Input: dimensioned drawing with shaded views. Units: mm. Origin: part minimum x, y, z. A direction names the side the tool comes from. Give positions to 0.01 mm unless a question says otherwise; leave off trailing zeros. Loops run counter-clockwise (first coordinate to the right, second up) from the corner with the lowest first, then second, coordinate; pieces in that order, holes last. Notation, with made-up numbers: (-19, 9) -> (16, 9) arc R21 cw to (16, 15) -> close; hole circle Ø7 at (-11, 32). An arc over 180 degrees is marked (long way). Answer as a JSON object with one key per item and string values.
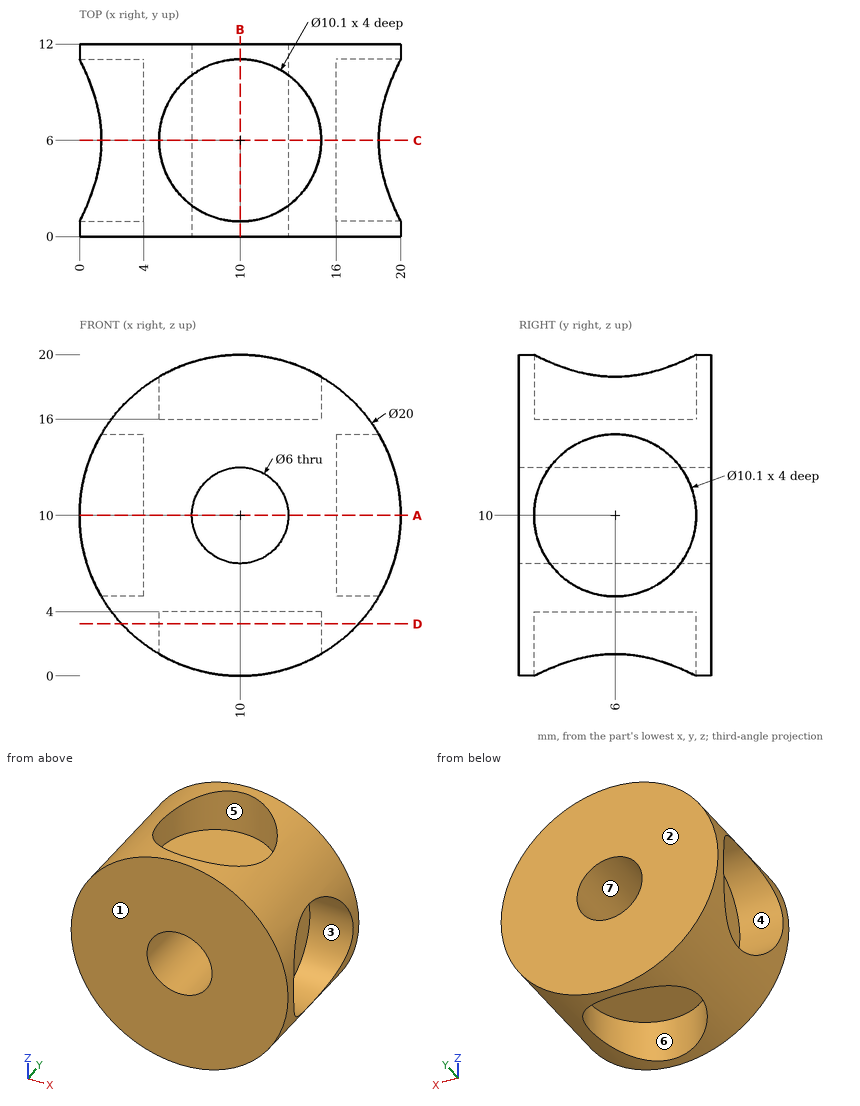
Q1. Section C-C, the plane y = 6. Return the cut outline in (x, z), then the cut area to 3 significant figures.
Evaluation:
{"outline": "(1.37, 4.95) arc R10 ccw to (4.95, 1.37) -> (4.95, 4) -> (15.05, 4) -> (15.05, 1.37) arc R10 ccw to (18.63, 4.95) -> (16, 4.95) -> (16, 15.05) -> (18.63, 15.05) arc R10 ccw to (15.05, 18.63) -> (15.05, 16) -> (4.95, 16) -> (4.95, 18.63) arc R10 ccw to (1.37, 15.05) -> (4, 15.05) -> (4, 4.95) -> close; hole circle Ø6 at (10, 10)", "area": "142 mm2"}
Q2. Section A-A, the plane z = 10. Return the cut outline in (x, y).
Evaluation:
{"outline": "(0, 0) -> (7, 0) -> (7, 12) -> (0, 12) -> (0, 11.05) -> (4, 11.05) -> (4, 0.95) -> (0, 0.95) -> close; (13, 0) -> (20, 0) -> (20, 0.95) -> (16, 0.95) -> (16, 11.05) -> (20, 11.05) -> (20, 12) -> (13, 12) -> close"}
Q3. Pin query (flat end, axial travel): pin 1 (7 mm diameter, centred on x = 10, z = 10, fed in from -Y); pin 2 (4 mm diameter, centred on y = 2, z = 17.5, fed in from -X); pin 3 (3 mm diameter, centred on y = 4.5, z = 9.5, fed in from -X); pin 4 (2 mm diameter, centred on x = 12.5, y = 5, fed in from -Z). Return the tip coordinate at first contact, or that it passes through.
Evaluation:
{"pin 1": "stops at y = 0", "pin 2": "stops at x = 1.65", "pin 3": "stops at x = 4", "pin 4": "stops at z = 4"}
Q4. Draft query along Y for the marked faces 1, 2 and 3. Return one class per face: +Y half, -Y half, draft (parallel to the pull), parting line (faces both ways), or undercut.
Evaluation:
{"face 1": "-Y half", "face 2": "+Y half", "face 3": "undercut"}
Q5. Section B-B, the plane x = 10. Return the cut outline in (y, z).
Evaluation:
{"outline": "(0, 0) -> (0.95, 0) -> (0.95, 4) -> (11.05, 4) -> (11.05, 0) -> (12, 0) -> (12, 7) -> (0, 7) -> close; (0, 13) -> (12, 13) -> (12, 20) -> (11.05, 20) -> (11.05, 16) -> (0.95, 16) -> (0.95, 20) -> (0, 20) -> close"}
Q6. Ray query, line 1 along X through (y, z) = (0.5, 10); line 2 along Y through (x, z) = (18.3, 10); line 3 along Z through (x, y) = (14, 7.75). Return the intervals inside material, ascending.
Evaluation:
{"line 1": "x = 0 to 7, 13 to 20", "line 2": "y = 0 to 0.95, 11.05 to 12", "line 3": "z = 4 to 16"}
Q7. Section D-D, the plane z = 3.25. Return the cut outline in (x, y), then the cut area to 3 significant figures.
Evaluation:
{"outline": "(2.62, 0) -> (17.38, 0) -> (17.38, 12) -> (2.62, 12) -> close; hole circle Ø10.1 at (10, 6)", "area": "97.0 mm2"}
Q8. Access query for the marked faces 4, 5, 6 and 7. Directions: +Z, -Z, +X, -X, +Y, -Y. A direction counts if a zero-diameter tool reaches every point of the face in a straight line with its end or side. Return the directions, or none.
Evaluation:
{"face 4": "-X", "face 5": "+Z", "face 6": "-Z", "face 7": "+Y, -Y"}
